```python
from build123d import *

# Parameters (mm, degrees)
SKETCH_1_W                   = 361
SKETCH_1_H                   = 12
EXTRUDE_1_DEPTH              = 8
CUT_EXTRUDE_1_DEPTH          = 362.072014978
CUT_EXTRUDE_2_DEPTH          = 362.072014978
CUT_EXTRUDE_3_DEPTH          = 362.072014978
CUT_EXTRUDE_4_DEPTH          = 362.072014978
CUT_EXTRUDE_5_DEPTH          = 362.072014978
CUT_EXTRUDE_6_DEPTH          = 362.072014978
HOLE_WIZARD_M3_1_D           = 3.5
HOLE_WIZARD_M3_1_CBORE_D     = 5.9999
HOLE_WIZARD_M3_1_CBORE_DEPTH = 4.5
CHAMFER_1_SIZE               = 0.6
FILLET_1_R                   = 0.2


with BuildPart() as part:
    # 草图1 → 凸台-拉伸1 (new body)
    with BuildSketch(Plane(origin=(0, 4, 0), x_dir=(1, 0, 0), z_dir=(0, 1, 0))):
        Rectangle(SKETCH_1_W, SKETCH_1_H)
    extrude(amount=-EXTRUDE_1_DEPTH)

    # 草图2 → 切除-拉伸1 (cut, through all)
    with BuildSketch(Plane(origin=(180.5, 0, 0), x_dir=(0, 0, -1), z_dir=(1, 0, 0))):
        with BuildLine():
            Line((6, 1.51), (6, 2.01))
            Line((6, 2.01), (4.8, 2.01))
            ThreePointArc((4.8, 2.01), (4.55, 1.76), (4.8, 1.51))
            Line((4.8, 1.51), (6, 1.51))
        make_face()
    extrude(amount=-CUT_EXTRUDE_1_DEPTH, mode=Mode.SUBTRACT)

    # 草图3 → 切除-拉伸2 (cut, through all)
    with BuildSketch(Plane(origin=(180.5, 0, 0), x_dir=(0, 0, -1), z_dir=(1, 0, 0))):
        with BuildLine():
            Line((6, 2.01), (6, 3.111111))
            ThreePointArc((6, 3.111111), (5.367595703, 2.693428684), (5.04, 2.01))
            Line((5.04, 2.01), (6, 2.01))
        make_face()
    extrude(amount=-CUT_EXTRUDE_2_DEPTH, mode=Mode.SUBTRACT)

    # 草图4 → 切除-拉伸3 (cut, through all)
    with BuildSketch(Plane(origin=(180.5, 0, 0), x_dir=(0, 0, -1), z_dir=(1, 0, 0))):
        with BuildLine():
            Line((6, 1.51), (5.04, 1.51))
            ThreePointArc((5.04, 1.51), (5.367595703, 0.826571316), (6, 0.408889))
            Line((6, 0.408889), (6, 1.51))
        make_face()
    extrude(amount=-CUT_EXTRUDE_3_DEPTH, mode=Mode.SUBTRACT)

    # 草图5 → 切除-拉伸4 (cut, through all)
    with BuildSketch(Plane(origin=(180.5, 0, 0), x_dir=(0, 0, -1), z_dir=(1, 0, 0))):
        with BuildLine():
            Line((-6, 2.01), (-6, 1.51))
            Line((-6, 1.51), (-4.8, 1.51))
            ThreePointArc((-4.8, 1.51), (-4.55, 1.76), (-4.8, 2.01))
            Line((-4.8, 2.01), (-6, 2.01))
        make_face()
    extrude(amount=-CUT_EXTRUDE_4_DEPTH, mode=Mode.SUBTRACT)

    # 草图6 → 切除-拉伸5 (cut, through all)
    with BuildSketch(Plane(origin=(180.5, 0, 0), x_dir=(0, 0, -1), z_dir=(1, 0, 0))):
        with BuildLine():
            Line((-6, 1.51), (-6, 0.408889))
            ThreePointArc((-6, 0.408889), (-5.367595703, 0.826571316), (-5.04, 1.51))
            Line((-5.04, 1.51), (-6, 1.51))
        make_face()
    extrude(amount=-CUT_EXTRUDE_5_DEPTH, mode=Mode.SUBTRACT)

    # 草图7 → 切除-拉伸6 (cut, through all)
    with BuildSketch(Plane(origin=(180.5, 0, 0), x_dir=(0, 0, -1), z_dir=(1, 0, 0))):
        with BuildLine():
            Line((-6, 2.01), (-5.04, 2.01))
            ThreePointArc((-5.04, 2.01), (-5.367595703, 2.693428684), (-6, 3.111111))
            Line((-6, 3.111111), (-6, 2.01))
        make_face()
    extrude(amount=-CUT_EXTRUDE_6_DEPTH, mode=Mode.SUBTRACT)

    # M3 六角头机械螺钉的柱形沉头孔1 (through all)
    with Locations(Plane(origin=(0, 4, 0), x_dir=(1, 0, 0), z_dir=(0, 1, 0))):
        with Locations((-175, 0), (-150, 0), (-125, 0), (-100, 0), (-75, 0), (-50, 0), (-25, 0), (0, 0), (25, 0), (50, 0), (75, 0), (100, 0), (125, 0), (150, 0), (175, 0)):
            CounterBoreHole(HOLE_WIZARD_M3_1_D / 2, HOLE_WIZARD_M3_1_CBORE_D / 2, HOLE_WIZARD_M3_1_CBORE_DEPTH)

    # 倒角1
    chamfer_1_edges = [part.edges().sort_by_distance(p)[0] for p in [
        (0, -4, -6),
        (0, -4, 6),
    ]]
    chamfer(chamfer_1_edges, length=CHAMFER_1_SIZE)

    # 圆角1
    fillet_1_edges = [part.edges().sort_by_distance(p)[0] for p in [
        (0, 2.01, -5.04),
        (0, 3.111111, -6),
        (0, 0.408889, -6),
        (0, 1.51, -5.04),
        (0, 4, -6),
        (0, 4, 6),
        (0, 1.51, 5.04),
        (0, 0.408889, 6),
        (0, 3.111111, 6),
        (0, 2.01, 5.04),
    ]]
    fillet(fillet_1_edges, radius=FILLET_1_R)


solid = part.part
```
Verification items for the finished model (mm, model axes). Round coordinates to 2 decimals unless told otherwise and drop trailing zeros. Write each loop counter-clockwise with the first axis right and the second up, starting at its lowest first coordinate (ties: lowest second). Pieces come first, ordered by that corner, then holes. Notation, with made-up numbers: (29, 44.25) -> (54, 44.25) arc R32 ccw to (54, 74.25) -> close; hole circle Ø10 at (53, -5.5). An arc over 180 degrees is marked (long way). Write each question's results on one line, items separated by ' | '. Start each with the question number.
1. Material ranges on probe 1 along Z at (x, y) = (150, -1.7); probe 2 along Z at (x, y) = (0, 0.45); probe 3 along Y at (x, z) = (5.5, 5.25), recorded low to high. Write a range as from..to.
2. Cross-section at A-A (y = -2). Count the separate pieces of the cut face and the enclosed holes in it, then the cut area to 3 significant figures.
3. Draft check along Z on faces 1 (the cylindrical face through (77.86, 1.78, -0.9)), 2 (the flat face through (-123, -0.5, 0)). Enter one of: +Z half, -Z half, draft (parallel to the pull), parting line (faces both ways), or undercut.
4. Cross-section at B-B (x = 106). Enter the section's corners in (y, z), then the cut area to 3 significant figures.
5. Depth check by flat-ended pin: P1, Ø1.8, axis at x = -123.5, z = 0, coming from the +Y side; P2, Ø3, axis at x = -75, z = 0, coming from the -Y side. Enter the tip coordinate at first touch or a pass-through.
Solutions:
1) probe 1: z = -6..-1.75, 1.75..6 | probe 2: z = -5.89..-3, 3..5.89 | probe 3: y = -4..0.98, 2.54..4
2) separate pieces: 1 | enclosed holes: 15 | area: 4,190 mm2
3) face 1: undercut | face 2: undercut
4) outline: (-4, -5.4) -> (-3.4, -6) -> (0.27, -6) arc R0.2 ccw to (0.45, -5.88) arc R1.42 cw to (1.37, -5.07) arc R0.2 ccw to (1.51, -4.88) -> (1.51, -4.8) arc R0.25 cw to (2.01, -4.8) -> (2.01, -4.88) arc R0.2 ccw to (2.15, -5.07) arc R1.42 cw to (3.07, -5.88) arc R0.2 ccw to (3.25, -6) -> (3.8, -6) arc R0.2 ccw to (4, -5.8) -> (4, 5.8) arc R0.2 ccw to (3.8, 6) -> (3.25, 6) arc R0.2 ccw to (3.07, 5.88) arc R1.42 cw to (2.15, 5.07) arc R0.2 ccw to (2.01, 4.88) -> (2.01, 4.8) arc R0.25 cw to (1.51, 4.8) -> (1.51, 4.88) arc R0.2 ccw to (1.37, 5.07) arc R1.42 cw to (0.45, 5.88) arc R0.2 ccw to (0.27, 6) -> (-3.4, 6) -> (-4, 5.4) -> close | area: 91.3 mm2
5) P1: stops at y = -0.5 | P2: passes through
